Verification items for this drawing (mm, ordinates from the low corner). A direction names the side the tool comes from. Coordinates: 2 decimals unless noted, no trailing zeros. Order: outer loops, then holes, each group sorted by start corner. A loop starts at its lowest first (then second) coordinate and runs counter-clockwise, first axis right, second up. Notation, with made-up numbers: (36.25, 9.25) -> (74.25, 9.25) arc R33 cw to (74.25, 47.25) -> close; hole circle Ø4 at (84, 49.5). An arc over 180 degrees is marked (long way). Answer as CSV lines item,"result". Start each with the question number.
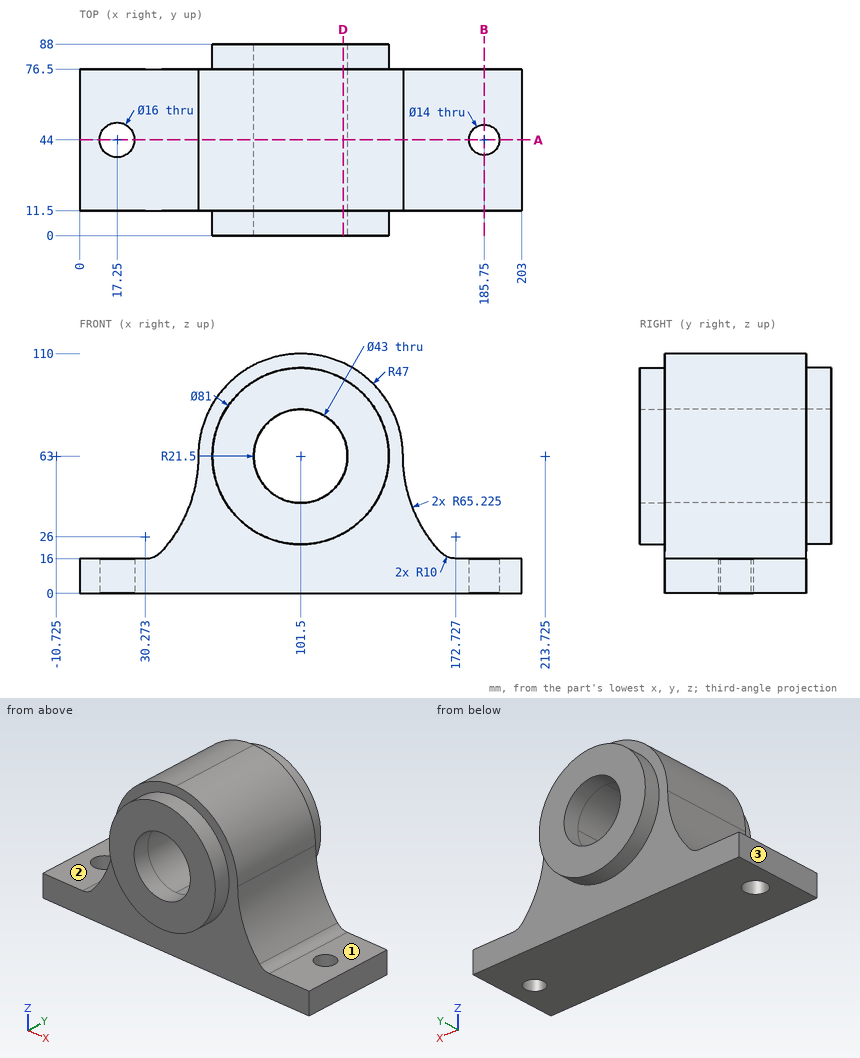
Q1. Thickness scan on L1, parallel to X at y = 66, z = 64; L2, parallel to Z at x = 101.5, y = 84; L3, parallel to Z at x = 16, y = 31. Record the ranges inside material, lowest first.
Q2. Sectioned sample at D-D, the plane x = 121. Record the cut outline in (y, z) (1 decimal), then the cut area to 3 significant figures.
Q3. Sectioned sample at A-A, the plane y = 44. Give the number of separate pieces and of enclosed holes in the cut face, then the cut area to 3 significant figures.
Q4. Sectioned sample at B-B, the plane x = 185.75. Record the cut outline in (y, z), then the cut area to 3 significant figures.
Q5. Access from +Z, -Z, +X, -X, +Y, -Y to the whole of each face (thin tool, end or side, straight path). Record for the marked faces 1, 2 and 3.
Q6. Go/stop test with flat-tipped pins: pin 1 Ø15 at (x, y) = (195, 55.5) entering from +Z; pin 2 Ø13 at (x, y) = (17.25, 44) entering from -Z; pin 3 Ø3 at (x, y) = (40, 40.5) entering from +Z (1 decimal); pin 4 Ø2 at (y, z) = (29, 26.5) entering from -X. Record where each tip stops, or that it passes through.
Geometry results:
1,L1,"x = 54.51 to 80.02, 122.98 to 148.49"
1,L2,"z = 22.5 to 41.5, 84.5 to 103.5"
1,L3,"z = 0 to 16"
2,outline,"(0, 27.5) -> (11.5, 27.5) -> (11.5, 0) -> (76.5, 0) -> (76.5, 27.5) -> (88, 27.5) -> (88, 53.9) -> (0, 53.9) -> close; (0, 72.1) -> (88, 72.1) -> (88, 98.5) -> (76.5, 98.5) -> (76.5, 105.8) -> (11.5, 105.8) -> (11.5, 98.5) -> (0, 98.5) -> close"
2,area,"6,910 mm^2"
3,separate pieces,"3"
3,enclosed holes,"1"
3,area,"9,790 mm^2"
4,outline,"(11.5, 0) -> (37, 0) -> (37, 16) -> (11.5, 16) -> close; (51, 0) -> (76.5, 0) -> (76.5, 16) -> (51, 16) -> close"
4,area,"816 mm^2"
5,face 1,"+Z, +X, +Y, -Y"
5,face 2,"+Z, -X, +Y, -Y"
5,face 3,"+Z, -Z, -X, +Y, -Y"
6,pin 1,"stops at z = 16"
6,pin 2,"passes through"
6,pin 3,"stops at z = 23.9"
6,pin 4,"stops at x = 42.64"
